Autodesk Inventor part; units mm, degrees
ref_plane "YZ Plane" through (0, 0, 0) normal (1, 0, 0) x (0, 1, 0)
ref_plane "XZ Plane" through (0, 0, 0) normal (0, 1, 0) x (-1, 0, 0)
ref_plane "XY Plane" through (0, 0, 0) normal (0, 0, 1) x (1, 0, 0)
sketch "Sketch1" plane through (0, 0, 0) normal (0, 0, 1) x (1, 0, 0)
  line L0 (10.5, 0) -> (21, 0) construction
  line L1 (10.5, 0) -> (21, 0) construction
  line L2 (21, 0) -> (21, -0.5)
  line L3 (21, -0.5) -> (20.5, -0.5)
  line L4 (20.5, -0.5) -> (20.5, -8.5)
  line L5 (20.5, -8.5) -> (21.5, -8.5)
  line L6 (21.5, -8.5) -> (21.5, 0)
  line L7 (21.5, 0) -> (21, 0)
  line L8 (10.5, 0) -> (10.5, -8) construction
  line L9 (10.5, 0) -> (18.5, 0) construction
  point P0 (0, 0)
  dimension "d1" = 0
  dimension "d2" = 0.5
  dimension "d3" = 90
  dimension "d4" = 0.5
  dimension "d5" = 270
  dimension "d6" = 8
  dimension "d7" = 1
  dimension "d8" = 8.5
  dimension "d9" = 8
  dimension "d10" = 90
  dimension "d11" = 10.5
revolve "Revolution1" add sketch "Sketch1" angle 360 about axis through (10.5, 0, 0) along (0, -1, 0)
fillet "Fillet1" radius 0.5 1 edges at (-0.5, -8.5, 0)
fillet "Fillet2" radius 0.25 1 edges at (-0.5, 0, 0)
properties part number "TIRE"
Model file for the job. Use its own axes, mm. Coordinates: 2 decimals unless noted, no trailing zeros. Write each loop counter-clockwise with the first axis right and the second up, starting at its lowest first coordinate (ties: lowest second). Pieces come first, ordered by that corner, then holes. Notation, with made-up numbers: (44, 74.25) - (86, 74.25) arc R14 ccw to (86, 90.25) - close; hole circle Ø3 at (12, 31). An arc over 180 degrees is marked (long way). Use a Markdown table: item, result. Add a question column.
Item 1: Band-saw the part on C-C, the plane y = -1. Write the cut outline in (x, z), and give its area (3 significant figures).
Item 2: Drop flat-ended pins along their axis: pin 1 (2 mm diameter, centred on x = 1.5, z = 8.5, fed in from +Y); pin 2 (2 mm diameter, centred on y = -7, z = 6.5, fed in from +X); pin 3 (1 mm diameter, centred on x = 4.5, y = -7.5, fed in from -Z); pin 4 (1 mm diameter, centred on y = -3.5, z = -2.5, fed in from +X). Give the stop position or say it passes through.
Item 3: Band-saw the part on A-A, the plane z = 0. Write the cut outline in (x, y), and give its area (3 significant figures).
Item 4: Band-saw the part on B-B, the plane x = 10.5. Write the cut outline in (y, z), and give its area (3 significant figures).
Item 5: Two-plate mould, pull along X, no slides. Class faces 1 (the face through (20.661, -4.071, 4.213)), 2 (the face through (20, -0.5, -4)), 3 (the face through (0.51, -4.56, 0.44)), 4 (the face through (20, -8.5, -4)): pulls with the +X half, pulls with the -X half, needs draft (parallel to the pull), parting line crosses it, or undercut.
Item 6: Drill centre lines: line 1 along Z through (x, y) = (10.5, -4); line 2 along Z through (x, y) = (10.5, -0.4); line 3 along X through (y, z) = (-1.25, -6.25). Where is each one in solid material? Low to high.
A:
| question | item | result |
|---|---|---|
| 1 | outline | circle Ø22 at (10.5, 0); hole circle Ø20 at (10.5, 0) |
| 1 | area | 66.0 mm² |
| 2 | pin 1 | passes through |
| 2 | pin 2 | stops at x = 20.03 |
| 2 | pin 3 | stops at z = -9.53 |
| 2 | pin 4 | stops at x = 21.32 |
| 3 | outline | (-0.5, -8) arc R0.5 ccw to (0, -8.5) - (0.5, -8.5) - (0.5, -0.5) - (0, -0.5) - (0, 0) - (-0.25, 0) arc R0.25 ccw to (-0.5, -0.25) - close; (20.5, -8.5) - (21, -8.5) arc R0.5 ccw to (21.5, -8) - (21.5, -0.25) arc R0.25 ccw to (21.25, 0) - (21, 0) - (21, -0.5) - (20.5, -0.5) - close |
| 3 | area | 16.4 mm² |
| 4 | outline | (-8.5, -10.5) arc R0.5 ccw to (-8, -11) - (-0.25, -11) arc R0.25 ccw to (0, -10.75) - (0, -10.5) - (-0.5, -10.5) - (-0.5, -10) - (-8.5, -10) - close; (-8.5, 10) - (-0.5, 10) - (-0.5, 10.5) - (0, 10.5) - (0, 10.75) arc R0.25 ccw to (-0.25, 11) - (-8, 11) arc R0.5 ccw to (-8.5, 10.5) - close |
| 4 | area | 16.4 mm² |
| 5 | face 1 | parting line crosses it |
| 5 | face 2 | undercut |
| 5 | face 3 | undercut |
| 5 | face 4 | needs draft |
| 6 | line 1 | z = -11 to -10, 10 to 11 |
| 6 | line 2 | z = -11 to -10.5, 10.5 to 11 |
| 6 | line 3 | x = 1.45 to 2.69, 18.31 to 19.55 |
